```python
from build123d import *

# Parameters (mm, degrees)
BOSS_EXTRUDE2_DEPTH = 15
CUT_EXTRUDE1_DEPTH  = 40.812058475


with BuildPart() as part:
    # Sketch5 → Boss-Extrude2 (new body)
    with BuildSketch(Plane(origin=(0, 0, 0), x_dir=(1, 0, 0), z_dir=(0, 1, 0))):
        with BuildLine():
            Line((0, 0), (32, 0))
            ThreePointArc((32, 0), (36, 4), (32, 8))
            Line((32, 8), (0, 8))
            ThreePointArc((0, 8), (-4, 4), (0, 0))
        make_face()
    extrude(amount=BOSS_EXTRUDE2_DEPTH)

    # Sketch8 → Cut-Extrude1 (cut, through all)
    with BuildSketch(Plane(origin=(0, 15, 0), x_dir=(1, 0, 0), z_dir=(0, 1, 0))):
        with BuildLine():
            Line((3, 5.8), (8, 5.8))
            ThreePointArc((8, 5.8), (9.8, 4), (8, 2.2))
            Line((8, 2.2), (3, 2.2))
            ThreePointArc((3, 2.2), (1.2, 4), (3, 5.8))
        make_face()
        with BuildLine():
            Line((25, 5.8), (30, 5.8))
            ThreePointArc((30, 5.8), (31.8, 4), (30, 2.2))
            Line((30, 2.2), (25, 2.2))
            ThreePointArc((25, 2.2), (23.2, 4), (25, 5.8))
        make_face()
    extrude(amount=-CUT_EXTRUDE1_DEPTH, mode=Mode.SUBTRACT)


solid = part.part
```
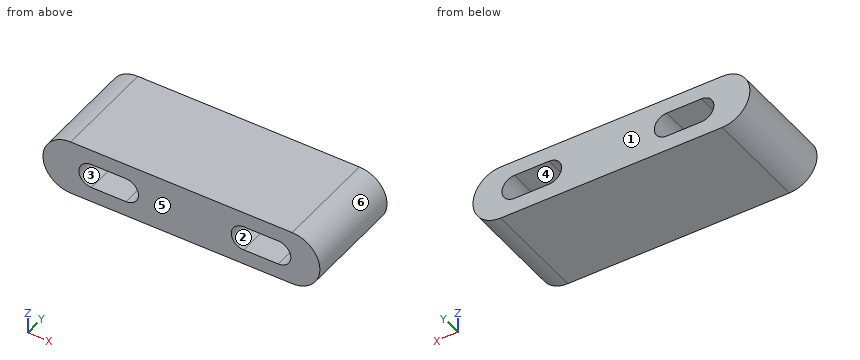
Design review of the part built by this model. Coordinates are the model's own, in mm. Face numbers are marked on the shaded views. A direction names the side the tool comes from. Round coordinates to 2 decimals unless told otherwise and drop trailing zeros. Order: outer loops, then holes, each group sorted by start corner. A loop starts at its lowest first (then second) coordinate and runs counter-clockwise, first axis right, second up. Notation, with made-up numbers: (25, 64) - (32, 64) arc R18 ccw to (32, 79) - close; hole circle Ø1 at (4, -35). An arc over 180 degrees is marked (long way). Return JSON: item names as keys, results as strings.
Q1. Consider section C-C on x = 2.5. Write out the cut boundary in (y, z).
Computed values:
{"outline": "(0, -8) - (15, -8) - (15, -5.73) - (0, -5.73) - close; (0, -2.27) - (15, -2.27) - (15, 0) - (0, 0) - close"}
Q2. Wall thickness on L1, parallel to X at y = 2, z = -4; L2, parallel to X at y = 14, z = -5; L3, parallel to Z at x = 25, y = 11.5: over which ranges is each line inside the solid? List them lowest first. Write a range as [from, to].
Computed values:
{"L1": "x = [-4, 1.2], [9.8, 23.2], [31.8, 36]", "L2": "x = [-3.87, 1.5], [9.5, 23.5], [31.5, 35.87]", "L3": "z = [-8, -5.8], [-2.2, 0]"}
Q3. Consider section B-B on z = -4. Write out the cut boundary in (x, y), plus the area to 3 significant figures.
Computed values:
{"outline": "(-4, 0) - (1.2, 0) - (1.2, 15) - (-4, 15) - close; (9.8, 0) - (23.2, 0) - (23.2, 15) - (9.8, 15) - close; (31.8, 0) - (36, 0) - (36, 15) - (31.8, 15) - close", "area": "342 mm2"}
Q4. Machinability: for the marked faces 1 and 2, which of the approach directions +Z, -Z, +X, -X, +Y, -Y give a long, thin tool a straight path to every point of the face, cutting with its end or side? Answer none if there is none.
Computed values:
{"face 1": "+Z, -Z, +X, -X, +Y", "face 2": "+Y, -Y"}
Q5. Consider section D-D on z = -1.5. Write out the cut boundary in (x, y).
Computed values:
{"outline": "(-3.12, 0) - (35.12, 0) - (35.12, 15) - (-3.12, 15) - close"}
Q6. Consider section A-A on y = 9.5. Write out the cut boundary in (x, z).
Computed values:
{"outline": "(0, -8) - (32, -8) arc R4 ccw to (32, 0) - (0, 0) arc R4 ccw to start; hole (3, -5.8) - (8, -5.8) arc R1.8 ccw to (8, -2.2) - (3, -2.2) arc R1.8 ccw to start; hole (25, -5.8) - (30, -5.8) arc R1.8 ccw to (30, -2.2) - (25, -2.2) arc R1.8 ccw to start"}
Q7. The part is to be moulded in two halves that separate along X. For the marked faces 3, 4, 5 and 6, say which applies: pulls with the +X half, pulls with the -X half, needs draft (parallel to the pull), parting line crosses it, or undercut.
Computed values:
{"face 3": "undercut", "face 4": "undercut", "face 5": "needs draft", "face 6": "pulls with the +X half"}
